Can you work these out from the model? Positions are in its coordinate system, mm. Face numbers are marked on the shaded views. A direction names the side the tool comes from. Coordinates: 2 decimals unless noted, no trailing zeros. Order: outer loops, then holes, each group sorted by start corner. A loop starts at its lowest first (then second) coordinate and runs counter-clockwise, first axis right, second up.
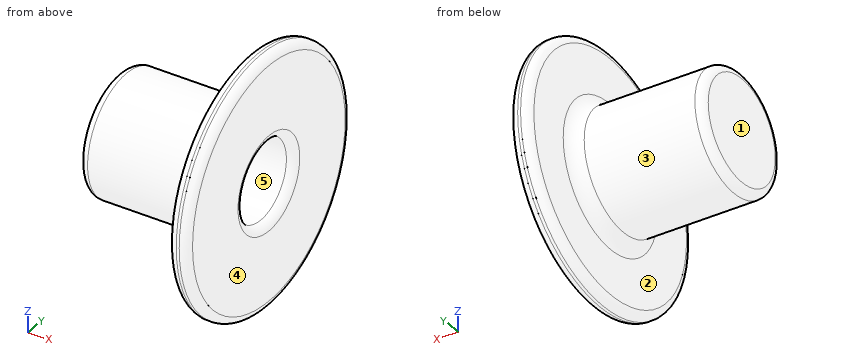
```python
from build123d import *


with BuildPart() as part:
    # 草图1 → 旋转1 (revolve)
    with BuildSketch(Plane.XY):
        with BuildLine():
            Line((-455, 8.382), (-455, 0.277))
            Line((-455, 0.277), (-450, 0.277))
            Line((-450, 0.277), (-450, 6.477))
            Line((-450, 6.477), (-432.612413979, 6.477))
            ThreePointArc((-432.612413979, 6.477), (-431.714388367, 6.848974388), (-431.342413979, 7.747))
            Line((-431.342413979, 7.747), (-431.342413979, 18.73))
            ThreePointArc((-431.342413979, 18.73), (-431.714388367, 19.628025612), (-432.612413979, 20))
            Line((-432.612413979, 20), (-433.072413979, 20))
            ThreePointArc((-433.072413979, 20), (-433.970439591, 19.628025612), (-434.342413979, 18.73))
            Line((-434.342413979, 18.73), (-434.342413979, 11.652))
            ThreePointArc((-434.342413979, 11.652), (-434.928200417, 10.237786438), (-436.342413979, 9.652))
            Line((-436.342413979, 9.652), (-453.73, 9.652))
            ThreePointArc((-453.73, 9.652), (-454.628025612, 9.280025612), (-455, 8.382))
        make_face()
    revolve(axis=Axis((-455.001250002, 0.277, 0), (1, 0, 0)))


solid = part.part
```
1. Imagine slicing it at A-A on z = 0. Please give me the cut outline in (x, y).
Completed:
outline: (-455, -7.83) arc R1.27 ccw to (-453.73, -9.1) - (-436.34, -9.1) arc R2 cw to (-434.34, -11.1) - (-434.34, -18.18) arc R1.27 ccw to (-433.07, -19.45) - (-432.61, -19.45) arc R1.27 ccw to (-431.34, -18.18) - (-431.34, -7.19) arc R1.27 ccw to (-432.61, -5.92) - (-450, -5.92) - (-450, 6.48) - (-432.61, 6.48) arc R1.27 ccw to (-431.34, 7.75) - (-431.34, 18.73) arc R1.27 ccw to (-432.61, 20) - (-433.07, 20) arc R1.27 ccw to (-434.34, 18.73) - (-434.34, 11.65) arc R2 cw to (-436.34, 9.65) - (-453.73, 9.65) arc R1.27 ccw to (-455, 8.38) - close
2. Imagine slicing it at B-B on x = -444. Please give me the cut outline in (y, z) (3 decimals).
Completed:
outline: circle Ø18.75 at (0.277, 0); hole circle Ø12.4 at (0.277, 0)
3. Please list where these lines run through material, in increasing order: probe 1 along X at (y, z) = (-13, -8.5); probe 2 along X at (y, z) = (-1.5, 1); probe 3 along Z at (x, y) = (-435.5, -1).
Completed:
probe 1: x = -434.34 to -431.34
probe 2: x = -455 to -450
probe 3: z = -9.48 to -6.07, 6.07 to 9.48
4. Thinking about a two-plate mould opening in Y: for the marked faces 3, 4 and 5, which applies, pulls with the +Y half, pulls with the -Y half, needs draft (parallel to the pull), parting line crosses it, or undercut?
Completed:
face 3: parting line crosses it
face 4: needs draft
face 5: undercut
5. I'm going to push flat-ended pins straight in: pin 1 (5 mm diameter, centred on x = -447, y = -7.5, fed in from +Z); pin 2 (3 mm diameter, centred on x = -443.5, z = -2, fed in from +Y); pin 3 (2 mm diameter, centred on x = -440.5, z = 0.5, fed in from -Y). Where does each tip first touch, or does it pass through?
Completed:
pin 1: stops at z = 7.75
pin 2: stops at y = 9.64
pin 3: stops at y = -9.1
6. On a 3-axis mill with a long thin cutter (end or side, diameter ignored), from which of +Z, -Z, +X, -X, +Y, -Y can I reach the whole of each face in a straight line? I mean the marked faces 1 and 2. Say none if no direction works.
Completed:
face 1: +Z, -Z, -X, +Y, -Y
face 2: -X
